For this review, take the finished solid that the model builds, in its own axes (mm). A direction names the side the tool comes from. Coordinates: 2 decimals unless noted, no trailing zeros. Write each loop counter-clockwise with the first axis right and the second up, starting at its lowest first coordinate (ties: lowest second). Pieces come first, ordered by that corner, then holes. Notation, with made-up numbers: (2.5, 27.5) -> (21.5, 27.5) arc R37 cw to (21.5, 65.5) -> close; hole circle Ø1 at (31.5, 1). An arc over 180 degrees is marked (long way). Put each result on its own line as item: value. Start each with the question number.
Item 1: For faces 1 (the flat face through (342.9, 250, 3)), 2 (the flat face through (-55, 431.8, 3)), list the 3-axis set-ups (+Z, -Z, +X, -X, +Y, -Y) from which the entire face can be reached by the end or side of a thin tool; tool diameter is ignored.
Item 2: To check wall thickness, follow L1, parallel to Y at x = -94.5, z = 100; L2, parallel to X at y = 460, z = -138.5; L3, parallel to X at y = 477, z = -142. State the ranges of each line that lie inside material, in increasing order.
Item 3: Consider section B-B on x = 268. Give the boundary of the cut face in (y, z).
Item 4: Consider section C-C on y = 454. Give the boundary of the cut face in (x, z), and give its area (3 significant figures).
Item 5: Consider section A-A on z = -27.5. Give the boundary of the cut face in (x, y), and give its area (3 significant figures).
```python
from build123d import *

# Parameters (mm, degrees)
SKETCH1_W           = 685.8
SKETCH1_H           = 431.8
BOSS_EXTRUDE1_DEPTH = 508
CUT_EXTRUDE1_DEPTH  = 432.8


with BuildPart() as part:
    # Sketch1 → Boss-Extrude1 (new body)
    with BuildSketch(Plane(origin=(0, 0, 0), x_dir=(1, 0, 0), z_dir=(0, 1, 0))):
        Rectangle(SKETCH1_W, SKETCH1_H)
    extrude(amount=BOSS_EXTRUDE1_DEPTH)

    # Sketch2 → Cut-Extrude1 (cut, through all)
    with BuildSketch(Plane.XY.offset(215.9)):
        Polygon((-342.9, 431.8), (241.3, 431.8), (292.1, 508), (-342.9, 508), align=None)
    extrude(amount=-CUT_EXTRUDE1_DEPTH, mode=Mode.SUBTRACT)


solid = part.part
```
Return value:
1. face 1: +Z, -Z, +X, +Y, -Y
1. face 2: +Z, -Z, -X, +Y
2. L1: 0 to 431.8
2. L2: 260.1 to 342.9
2. L3: 271.43 to 342.9
3. outline: (0, -215.9) -> (471.85, -215.9) -> (471.85, 215.9) -> (0, 215.9) -> close
4. outline: (256.1, -215.9) -> (342.9, -215.9) -> (342.9, 215.9) -> (256.1, 215.9) -> close
4. area: 37,500 mm^2
5. outline: (-342.9, 0) -> (342.9, 0) -> (342.9, 508) -> (292.1, 508) -> (241.3, 431.8) -> (-342.9, 431.8) -> close
5. area: 302,000 mm^2
